Source: CAD feature listing. Evaluate the final solid. Frame: model axes, mm. Round coordinates to 2 decimals unless told otherwise and drop trailing zeros. Loops run counter-clockwise (first coordinate to the right, second up) from the corner with the lowest first, then second, coordinate; pieces in that order, holes last. Notation, with made-up numbers: (-33, 25) - (12, 25) arc R26 cw to (12, 64) - close; hole circle Ø6 at (50.25, 44). An arc over 180 degrees is marked (long way). One line per question, with ' | ' between items.
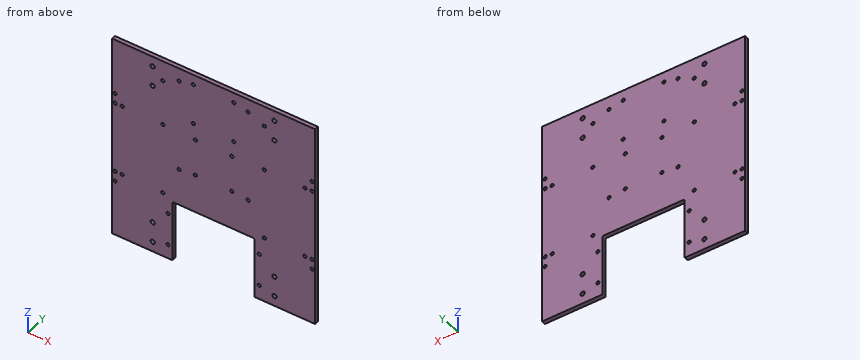
from build123d import *

# Parameters (mm, degrees)
SKETCH_1_W          = 200
SKETCH_1_H          = 200
SKETCH_1_R          = 1.6
SKETCH_1_R_2        = 2.1
EXTRUDE_1_DEPTH     = 4
CUT_EXTRUDE_1_REACH = 143.478
SKETCH_2_R          = 1.6
SKETCH_2_W          = 80.5
SKETCH_2_H          = 60
CUT_EXTRUDE_START   = -4
SKETCH_3_R          = 1.6
CUT_EXTRUDE_2_DEPTH = 4
FILLET_1_R          = 1


with BuildPart() as part:
    # 草图1 → 凸台-拉伸1 (new body)
    with BuildSketch(Plane(origin=(0, 0, 0), x_dir=(1, 0, 0), z_dir=(0, 1, 0))):
        Rectangle(SKETCH_1_W, SKETCH_1_H)
        with Locations(Location((-97, 35, 0), (0, 0, 270))):
            Circle(SKETCH_1_R, mode=Mode.SUBTRACT)
        with Locations(Location((-97, 45, 0), (0, 0, 270))):
            Circle(SKETCH_1_R, mode=Mode.SUBTRACT)
        with Locations(Location((-97, -45, 0), (0, 0, 90))):
            Circle(SKETCH_1_R, mode=Mode.SUBTRACT)
        with Locations(Location((-97, -35, 0), (0, 0, 90))):
            Circle(SKETCH_1_R, mode=Mode.SUBTRACT)
        with Locations(Location((97, -45, 0), (0, 0, 270))):
            Circle(SKETCH_1_R, mode=Mode.SUBTRACT)
        with Locations(Location((97, -35, 0), (0, 0, 270))):
            Circle(SKETCH_1_R, mode=Mode.SUBTRACT)
        with Locations(Location((97, 35, 0), (0, 0, 90))):
            Circle(SKETCH_1_R, mode=Mode.SUBTRACT)
        with Locations(Location((97, 45, 0), (0, 0, 90))):
            Circle(SKETCH_1_R, mode=Mode.SUBTRACT)
        with Locations(Location((-18, -34, 0), (0, 0, 270))):
            Circle(SKETCH_1_R, mode=Mode.SUBTRACT)
        with Locations(Location((18, -34, 0), (0, 0, 270))):
            Circle(SKETCH_1_R, mode=Mode.SUBTRACT)
        with Locations(Location((18, 2, 0), (0, 0, 270))):
            Circle(SKETCH_1_R, mode=Mode.SUBTRACT)
        with Locations(Location((-18, 2, 0), (0, 0, 270))):
            Circle(SKETCH_1_R, mode=Mode.SUBTRACT)
        with Locations(Location((-34, -87, 0), (0, 0, 270))):
            Circle(SKETCH_1_R, mode=Mode.SUBTRACT)
        with Locations(Location((34, -87, 0), (0, 0, 270))):
            Circle(SKETCH_1_R, mode=Mode.SUBTRACT)
        with Locations(Location((34, 3.6, 0), (0, 0, 270))):
            Circle(SKETCH_1_R, mode=Mode.SUBTRACT)
        with Locations(Location((-34, 3.6, 0), (0, 0, 270))):
            Circle(SKETCH_1_R, mode=Mode.SUBTRACT)
        with Locations(Location((-60, 90, 0), (0, 0, 270))):
            Circle(SKETCH_1_R_2, mode=Mode.SUBTRACT)
        with Locations(Location((-60, 70, 0), (0, 0, 270))):
            Circle(SKETCH_1_R_2, mode=Mode.SUBTRACT)
        with Locations(Location((60, 70, 0), (0, 0, 90))):
            Circle(SKETCH_1_R_2, mode=Mode.SUBTRACT)
        with Locations(Location((60, 90, 0), (0, 0, 90))):
            Circle(SKETCH_1_R_2, mode=Mode.SUBTRACT)
        with Locations(Location((60, -70, 0), (0, 0, 270))):
            Circle(SKETCH_1_R_2, mode=Mode.SUBTRACT)
        with Locations(Location((60, -90, 0), (0, 0, 270))):
            Circle(SKETCH_1_R_2, mode=Mode.SUBTRACT)
        with Locations(Location((-60, -70, 0), (0, 0, 90))):
            Circle(SKETCH_1_R_2, mode=Mode.SUBTRACT)
        with Locations(Location((-60, -90, 0), (0, 0, 90))):
            Circle(SKETCH_1_R_2, mode=Mode.SUBTRACT)
        with Locations(Location((-90, 35, 0), (0, 0, 270))):
            Circle(SKETCH_1_R, mode=Mode.SUBTRACT)
        with Locations(Location((-50, 35, 0), (0, 0, 270))):
            Circle(SKETCH_1_R, mode=Mode.SUBTRACT)
        with Locations(Location((-50, -35, 0), (0, 0, 270))):
            Circle(SKETCH_1_R, mode=Mode.SUBTRACT)
        with Locations(Location((-90, -35, 0), (0, 0, 270))):
            Circle(SKETCH_1_R, mode=Mode.SUBTRACT)
        with Locations(Location((90, 35, 0), (0, 0, 90))):
            Circle(SKETCH_1_R, mode=Mode.SUBTRACT)
        with Locations(Location((50, 35, 0), (0, 0, 90))):
            Circle(SKETCH_1_R, mode=Mode.SUBTRACT)
        with Locations(Location((50, -35, 0), (0, 0, 90))):
            Circle(SKETCH_1_R, mode=Mode.SUBTRACT)
        with Locations(Location((90, -35, 0), (0, 0, 90))):
            Circle(SKETCH_1_R, mode=Mode.SUBTRACT)
        with Locations(Location((-20, -50, 0), (0, 0, 270))):
            Circle(SKETCH_1_R, mode=Mode.SUBTRACT)
        with Locations(Location((20, -50, 0), (0, 0, 270))):
            Circle(SKETCH_1_R, mode=Mode.SUBTRACT)
        with Locations(Location((20, -90, 0), (0, 0, 270))):
            Circle(SKETCH_1_R, mode=Mode.SUBTRACT)
        with Locations(Location((-20, -90, 0), (0, 0, 270))):
            Circle(SKETCH_1_R, mode=Mode.SUBTRACT)
    extrude(amount=EXTRUDE_1_DEPTH)

    # 草图2 → 切除-拉伸1 (cut, up to next)
    with BuildSketch(Plane(origin=(0, 4, 0), x_dir=(1, 0, 0), z_dir=(0, 1, 0)), mode=Mode.PRIVATE) as cut_extrude_1_sk1:
        with Locations(Location((45, 86, 0), (0, 0, 270))):
            Circle(SKETCH_2_R)
    cut_extrude_1_tool1 = extrude(cut_extrude_1_sk1.sketch, amount=-CUT_EXTRUDE_1_REACH, mode=Mode.PRIVATE) & part.part
    # 草图2 → 切除-拉伸1 (cut, up to next)
    with BuildSketch(Plane(origin=(0, 4, 0), x_dir=(1, 0, 0), z_dir=(0, 1, 0)), mode=Mode.PRIVATE) as cut_extrude_1_sk2:
        with Locations(Location((45, 54, 0), (0, 0, 90))):
            Circle(SKETCH_2_R)
    cut_extrude_1_tool2 = extrude(cut_extrude_1_sk2.sketch, amount=-CUT_EXTRUDE_1_REACH, mode=Mode.PRIVATE) & part.part
    # 草图2 → 切除-拉伸1 (cut, up to next)
    with BuildSketch(Plane(origin=(0, 4, 0), x_dir=(1, 0, 0), z_dir=(0, 1, 0)), mode=Mode.PRIVATE) as cut_extrude_1_sk3:
        with Locations(Location((-45, 54, 0), (0, 0, 270))):
            Circle(SKETCH_2_R)
    cut_extrude_1_tool3 = extrude(cut_extrude_1_sk3.sketch, amount=-CUT_EXTRUDE_1_REACH, mode=Mode.PRIVATE) & part.part
    # 草图2 → 切除-拉伸1 (cut, up to next)
    with BuildSketch(Plane(origin=(0, 4, 0), x_dir=(1, 0, 0), z_dir=(0, 1, 0)), mode=Mode.PRIVATE) as cut_extrude_1_sk4:
        with Locations(Location((-45, 86, 0), (0, 0, 90))):
            Circle(SKETCH_2_R)
    cut_extrude_1_tool4 = extrude(cut_extrude_1_sk4.sketch, amount=-CUT_EXTRUDE_1_REACH, mode=Mode.PRIVATE) & part.part
    # 草图2 → 切除-拉伸1 (cut, up to next)
    with BuildSketch(Plane(origin=(0, 4, 0), x_dir=(1, 0, 0), z_dir=(0, 1, 0)), mode=Mode.PRIVATE) as cut_extrude_1_sk5:
        with Locations((0, 70)):
            Rectangle(SKETCH_2_W, SKETCH_2_H)
    cut_extrude_1_tool5 = extrude(cut_extrude_1_sk5.sketch, amount=-CUT_EXTRUDE_1_REACH, mode=Mode.PRIVATE) & part.part
    add(cut_extrude_1_tool1.solids().sort_by_distance((45, 4, -86))[0], mode=Mode.SUBTRACT)
    add(cut_extrude_1_tool2.solids().sort_by_distance((45, 4, -54))[0], mode=Mode.SUBTRACT)
    add(cut_extrude_1_tool3.solids().sort_by_distance((-45, 4, -54))[0], mode=Mode.SUBTRACT)
    add(cut_extrude_1_tool4.solids().sort_by_distance((-45, 4, -86))[0], mode=Mode.SUBTRACT)
    add(cut_extrude_1_tool5.solids().sort_by_distance((0, 4, -70))[0], mode=Mode.SUBTRACT)

    # 草图3 → 切除-拉伸2 (cut)
    with BuildSketch(Plane(origin=(0, 4, 0), x_dir=(1, 0, 0), z_dir=(0, 1, 0)).offset(CUT_EXTRUDE_START)):
        with Locations(Location((-50, -80, 0), (0, 0, 270))):
            Circle(SKETCH_3_R)
        with Locations(Location((50, -80, 0), (0, 0, 270))):
            Circle(SKETCH_3_R)
        with Locations(Location((50, 35, 0), (0, 0, 90))):
            Circle(SKETCH_3_R)
        with Locations(Location((-50, 35, 0), (0, 0, 270))):
            Circle(SKETCH_3_R)
    extrude(amount=CUT_EXTRUDE_2_DEPTH, mode=Mode.SUBTRACT)

    # 圆角1
    fillet_1_edges = [part.edges().sort_by_distance(p)[0] for p in [
        (40.25, 2, -100),
        (40.25, 2, -40),
        (-40.25, 2, -40),
        (-40.25, 2, -100),
    ]]
    fillet(fillet_1_edges, radius=FILLET_1_R)


solid = part.part
1. Section query B-B, the plane x = -12. Return loops of the section in (y, z).
Worked out:
outline: (0, -40) - (4, -40) - (4, 100) - (0, 100) - close
2. Section query A-A, the plane y = 1.05. Give the number of separate pieces and of enclosed holes in the cut face, plus the area to 3 significant figures.
Worked out:
separate pieces: 1 | enclosed holes: 42 | area: 34,800 mm2
3. Material intervals for probe 1 along X at (y, z) = (1.95, 70); probe 2 along Z at (x, y) = (-97, 1.2); probe 3 along X at (y, z) = (1.8, -70), sorted ascending.
Worked out:
probe 1: x = -100 to -62.1, -57.9 to 57.9, 62.1 to 100 | probe 2: z = -100 to -46.6, -43.4 to -36.6, -33.4 to 33.4, 36.6 to 43.4, 46.6 to 100 | probe 3: x = -100 to -62.1, -57.9 to -40.25, 40.25 to 57.9, 62.1 to 100
4. Contact query for a flat-ended pin moving along its axis: P1, Ø1.2, axis at x = -12.5, y = 3, coming from the -Z side. Output: stop coordinate, or through.
Worked out:
P1: stops at z = -40
